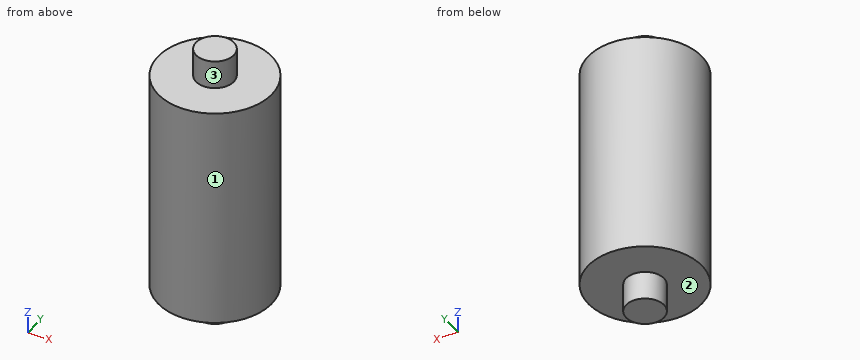
```python
from build123d import *

# Parameters (mm, degrees)
SKETCH1_R           = 15
BOSS_EXTRUDE1_DEPTH = 29.5
SKETCH2_R           = 5
BOSS_EXTRUDE2_DEPTH = 7.5
SKETCH3_R           = 5
BOSS_EXTRUDE3_DEPTH = 7.5


with BuildPart() as part:
    # Sketch1 → Boss-Extrude1 (new, symmetric)
    with BuildSketch(Plane.XY):
        Circle(SKETCH1_R)
    extrude(amount=BOSS_EXTRUDE1_DEPTH, both=True)

    # Sketch2 → Boss-Extrude2 (add, symmetric)
    with BuildSketch(Plane.XY.offset(29.5)):
        Circle(SKETCH2_R)
    extrude(amount=BOSS_EXTRUDE2_DEPTH, both=True)

    # Sketch3 → Boss-Extrude3 (add, symmetric)
    with BuildSketch(Plane(origin=(0, 0, -29.5), x_dir=(-1, 0, 0), z_dir=(0, 0, -1))):
        with Locations(Location((0, 0, 0), (0, 0, 180))):
            Circle(SKETCH3_R)
    extrude(amount=BOSS_EXTRUDE3_DEPTH, both=True)


solid = part.part
```
Work out the finished part from the listing and answer in its coordinate system (mm). Face numbers are marked on the shaded views. A direction names the side the tool comes from. Round coordinates to 2 decimals unless told otherwise and drop trailing zeros. Loops run counter-clockwise (first coordinate to the right, second up) from the corner with the lowest first, then second, coordinate; pieces in that order, holes last. Notation, with made-up numbers: M 33,45 L 38,45 A16 cw 38,65 Z; hole C 87,80 d2. An arc over 180 degrees is marked long. One line per question, with ' | ' between items.
Q1. Each of these flat-tipped pins is pushed along its axis until it touches: pin 1 Ø3 at (y, z) = (8, -28.5) entering from -X; pin 2 Ø10 at (x, z) = (-9.5, -17.5) entering from -Y; pin 3 Ø2 at (y, z) = (-9.5, 4) entering from -X. Where does it stop, or does it pass through?
Conclusion:
pin 1: stops at x = -13.52 | pin 2: stops at y = -14.31 | pin 3: stops at x = -12.36
Q2. Find section C-C, the plane z = 18.5. Give the vertices of the cut face in (x, y).
Conclusion:
outline: C 0,0 d30
Q3. Find section D-D, the plane y = 9. Give the vertices of the cut face in (x, z), then the cut area to 3 significant figures.
Conclusion:
outline: M -12,-29.5 L 12,-29.5 L 12,29.5 L -12,29.5 Z | area: 1,420 mm2
Q4. Find section A-A, the plane y = 0. Give the vertices of the cut face in (x, z), then the cut area to 3 significant figures.
Conclusion:
outline: M -15,-29.5 L -5,-29.5 L -5,-37 L 5,-37 L 5,-29.5 L 15,-29.5 L 15,29.5 L 5,29.5 L 5,37 L -5,37 L -5,29.5 L -15,29.5 Z | area: 1,920 mm2
Q5. Consider line 1 along Z through (x, y) = (-1.5, -12); line 2 along Y through (x, z) = (0, 2.5); line 3 along X through (y, z) = (1, -20.5). Determine where each line is inside the solid, lowest interval first. Write a range as from..to.
Conclusion:
line 1: z = -29.5..29.5 | line 2: y = -15..15 | line 3: x = -14.97..14.97
Q6. A tool of negligible diameter and unlimited length cuts with its end or side. For the marked faces 1, 2 and 3, from which of +Z, -Z, +X, -X, +Y, -Y can it reach the whole face along a straight path? Write none if from no direction.
Conclusion:
face 1: +Z, -Z | face 2: -Z | face 3: +Z
